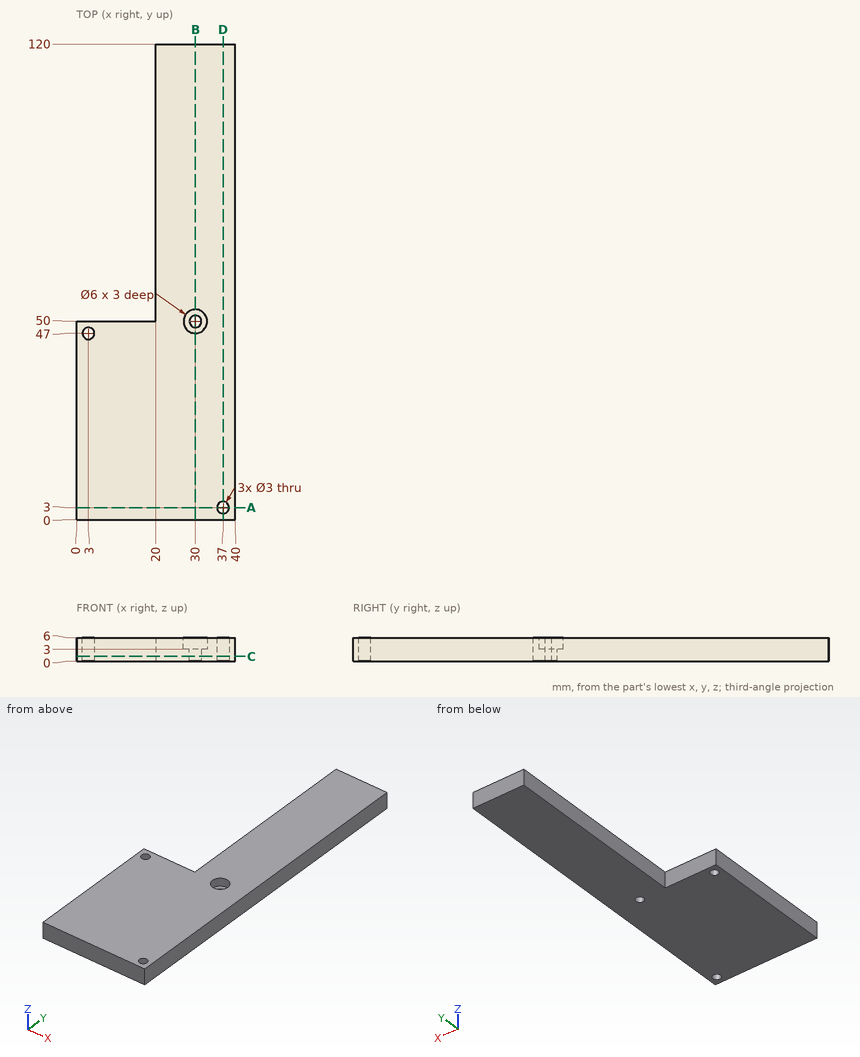
Source: three-view drawing plus pictorial views. Frame: mm from the lowest corner of the part. Round coordinates to 2 decimals unless told otherwise and drop trailing zeros. Loops run counter-clockwise (first coordinate to the right, second up) from the corner with the lowest first, then second, coordinate; pieces in that order, holes last.
Item 1: Section B-B, the plane x = 30. Output: boundary loops of the cut face in (y, z), plus the area to 3 significant figures.
Checked values:
outline: (0, 0) - (48.5, 0) - (48.5, 3) - (47, 3) - (47, 6) - (0, 6) - close; (51.5, 0) - (120, 0) - (120, 6) - (53, 6) - (53, 3) - (51.5, 3) - close
area: 693 mm2
Item 2: Section D-D, the plane x = 37. Output: boundary loops of the cut face in (y, z).
Checked values:
outline: (0, 0) - (1.5, 0) - (1.5, 6) - (0, 6) - close; (4.5, 0) - (120, 0) - (120, 6) - (4.5, 6) - close
Item 3: Section A-A, the plane y = 3. Output: boundary loops of the cut face in (x, z).
Checked values:
outline: (0, 0) - (35.5, 0) - (35.5, 6) - (0, 6) - close; (38.5, 0) - (40, 0) - (40, 6) - (38.5, 6) - close
Item 4: Section C-C, the plane z = 1.25. Output: boundary loops of the cut face in (x, y), plus the area to 3 significant figures.
Checked values:
outline: (0, 0) - (40, 0) - (40, 120) - (20, 120) - (20, 50) - (0, 50) - close; hole circle Ø3 at (3, 47); hole circle Ø3 at (30, 50); hole circle Ø3 at (37, 3)
area: 3,380 mm2
Item 5: Contact query for flat-ended pins moving along their axis: P1, Ø4, axis at x = 3, y = 47, coming from the -Z side; P2, Ø3, axis at x = 6.5, z = 2.5, coming from the +Y side; P3, Ø3, axis at x = 30, y = 50.5, coming from the +Z side; P4, Ø3, axis at y = 82, z = 3, coming from the -X side. Output: stop coordinate, or through.
Checked values:
P1: stops at z = 0
P2: stops at y = 50
P3: stops at z = 3
P4: stops at x = 20
Item 6: Line query: L1, parallel to Y at x = 30, z = 1.55; L2, parallel to Y at x = 3, z = 3.2; L3, parallel to Y at x = 6, z = 2.3. Output: solid intervals per line, ascending.
Checked values:
L1: y = 0 to 48.5, 51.5 to 120
L2: y = 0 to 45.5, 48.5 to 50
L3: y = 0 to 50
